```python
from build123d import *

# Parameters (mm, degrees)
SKETCH1_R           = 3.5
BOSS_EXTRUDE1_DEPTH = 60
BOSS_EXTRUDE2_DEPTH = 5
BOSS_EXTRUDE3_START = 5
SKETCH1_4_R         = 1.25
SKETCH1_4_R_2       = 2.143
BOSS_EXTRUDE3_DEPTH = 3
CUT_EXTRUDE1_REACH  = 213.819
BOSS_EXTRUDE4_START = 57
SKETCH1_6_R         = 3.5
SKETCH1_6_R_2       = 1.8
BOSS_EXTRUDE4_DEPTH = 3


with BuildPart() as part:
    # Sketch1 → Boss-Extrude1 (new body)
    with BuildSketch(Plane(origin=(0, 0, 0), x_dir=(1, 0, 0), z_dir=(0, 1, 0))):
        with BuildLine():
            ThreePointArc((0, 58.25), (17.061029996, 17.061029996), (58.25, 0))
            Line((58.25, 0), (118.99047, 0))
            ThreePointArc((118.99047, 0), (137.127758937, 7.512711063), (144.64047, 25.65))
            Line((144.64047, 25.65), (144.64047, 86.39047))
            ThreePointArc((144.64047, 86.39047), (127.579440004, 127.579440004), (86.39047, 144.64047))
            Line((86.39047, 144.64047), (58.25, 144.64047))
            ThreePointArc((58.25, 144.64047), (17.061029996, 127.579440004), (0, 86.39047))
            Line((0, 86.39047), (0, 58.25))
        make_face()
        with Locations(Location((66.320235, 6, 0), (0, 0, 270))):
            Circle(SKETCH1_R, mode=Mode.SUBTRACT)
        with BuildLine():
            ThreePointArc((5, 86.39047), (20.596563902, 124.043906098), (58.25, 139.64047))
            Line((58.25, 139.64047), (72.320235, 139.64047))
            Line((72.320235, 139.64047), (72.320235, 138.64047))
            ThreePointArc((72.320235, 138.64047), (78.320235, 132.64047), (84.320235, 138.64047))
            Line((84.320235, 138.64047), (84.320235, 139.600211843))
            ThreePointArc((84.320235, 139.600211843), (123.304711738, 124.768865705), (139.64047, 86.39047))
            Line((139.64047, 86.39047), (139.64047, 72.320235))
            Line((139.64047, 72.320235), (138.64047, 72.320235))
            ThreePointArc((138.64047, 72.320235), (132.64047, 66.320235), (138.64047, 60.320235))
            Line((138.64047, 60.320235), (139.64047, 60.320235))
            Line((139.64047, 60.320235), (139.64047, 25.65))
            ThreePointArc((139.64047, 25.65), (133.592225032, 11.048244968), (118.99047, 5))
            Line((118.99047, 5), (101.050235, 5))
            Line((101.050235, 5), (101.050235, 4.54))
            Line((101.050235, 4.54), (101.050235, 2))
            Line((101.050235, 2), (100.050235, 2))
            Line((100.050235, 2), (93.970235, 2))
            Line((93.970235, 2), (83.270235, 2))
            Line((83.270235, 2), (77.190235, 2))
            Line((77.190235, 2), (76.190235, 2))
            Line((76.190235, 2), (76.190235, 4.54))
            Line((76.190235, 4.54), (76.190235, 5))
            Line((76.190235, 5), (72.320235, 5))
            Line((72.320235, 5), (72.320235, 6))
            ThreePointArc((72.320235, 6), (66.320235, 12), (60.320235, 6))
            Line((60.320235, 6), (60.320235, 5))
            Line((60.320235, 5), (58.25, 5))
            ThreePointArc((58.25, 5), (20.596563902, 20.596563902), (5, 58.25))
            Line((5, 58.25), (5, 72.320235))
            Line((5, 72.320235), (6, 72.320235))
            ThreePointArc((6, 72.320235), (12, 78.320235), (6, 84.320235))
            Line((6, 84.320235), (5, 84.320235))
            Line((5, 84.320235), (5, 86.39047))
        make_face(mode=Mode.SUBTRACT)
        with Locations(Location((138.64047, 66.320235, 0), (0, 0, 270))):
            Circle(SKETCH1_R, mode=Mode.SUBTRACT)
        with Locations(Location((6, 78.320235, 0), (0, 0, 270))):
            Circle(SKETCH1_R, mode=Mode.SUBTRACT)
        with Locations(Location((78.320235, 138.64047, 0), (0, 0, 270))):
            Circle(SKETCH1_R, mode=Mode.SUBTRACT)
    extrude(amount=BOSS_EXTRUDE1_DEPTH)

    # Sketch1<2> → Boss-Extrude2 (add)
    with BuildSketch(Plane(origin=(0, 0, 0), x_dir=(1, 0, 0), z_dir=(0, 1, 0))):
        with BuildLine():
            Line((72.320235, 139.64047), (58.25, 139.64047))
            ThreePointArc((58.25, 139.64047), (20.596563902, 124.043906098), (5, 86.39047))
            Line((5, 86.39047), (5, 84.320235))
            Line((5, 84.320235), (6, 84.320235))
            ThreePointArc((6, 84.320235), (12, 78.320235), (6, 72.320235))
            Line((6, 72.320235), (5, 72.320235))
            Line((5, 72.320235), (5, 58.25))
            ThreePointArc((5, 58.25), (20.596563902, 20.596563902), (58.25, 5))
            Line((58.25, 5), (60.320235, 5))
            Line((60.320235, 5), (60.320235, 6))
            ThreePointArc((60.320235, 6), (66.320235, 12), (72.320235, 6))
            Line((72.320235, 6), (72.320235, 5))
            Line((72.320235, 5), (76.190235, 5))
            Line((76.190235, 5), (76.190235, 2))
            Line((76.190235, 2), (101.050235, 2))
            Line((101.050235, 2), (101.050235, 5))
            Line((101.050235, 5), (118.99047, 5))
            ThreePointArc((118.99047, 5), (133.592225032, 11.048244968), (139.64047, 25.65))
            Line((139.64047, 25.65), (139.64047, 60.320235))
            Line((139.64047, 60.320235), (138.64047, 60.320235))
            ThreePointArc((138.64047, 60.320235), (132.64047, 66.320235), (138.64047, 72.320235))
            Line((138.64047, 72.320235), (139.64047, 72.320235))
            Line((139.64047, 72.320235), (139.64047, 86.39047))
            ThreePointArc((139.64047, 86.39047), (123.304711738, 124.768865705), (84.320235, 139.600211843))
            Line((84.320235, 139.600211843), (84.320235, 138.64047))
            ThreePointArc((84.320235, 138.64047), (78.320235, 132.64047), (72.320235, 138.64047))
            Line((72.320235, 138.64047), (72.320235, 139.64047))
        make_face()
    extrude(amount=BOSS_EXTRUDE2_DEPTH)

    # Sketch1<4> → Boss-Extrude3 (add)
    # profile 1 of 4: a face of its own
    with BuildSketch(Plane(origin=(0, 0, 0), x_dir=(1, 0, 0), z_dir=(0, 1, 0)).offset(BOSS_EXTRUDE3_START)):
        with BuildLine():
            Line((101.050235, 2), (101.050235, 4.54))
            ThreePointArc((101.050235, 4.54), (97.510235, 8.08), (93.970235, 4.54))
            Line((93.970235, 4.54), (93.970235, 2))
            Line((93.970235, 2), (101.050235, 2))
        make_face()
        with Locations(Location((97.510235, 4.54, 0), (0, 0, 270))):
            Circle(SKETCH1_4_R, mode=Mode.SUBTRACT)
    # profile 2 of 4: a face of its own
    with BuildSketch(Plane(origin=(0, 0, 0), x_dir=(1, 0, 0), z_dir=(0, 1, 0)).offset(BOSS_EXTRUDE3_START)):
        with BuildLine():
            ThreePointArc((83.270235, 4.54), (79.730235, 8.08), (76.190235, 4.54))
            Line((76.190235, 4.54), (76.190235, 2))
            Line((76.190235, 2), (83.270235, 2))
            Line((83.270235, 2), (83.270235, 4.54))
        make_face()
        with Locations(Location((79.730235, 4.54, 0), (0, 0, 270))):
            Circle(SKETCH1_4_R, mode=Mode.SUBTRACT)
    # profile 3 of 4: a face of its own
    with BuildSketch(Plane(origin=(0, 0, 0), x_dir=(1, 0, 0), z_dir=(0, 1, 0)).offset(BOSS_EXTRUDE3_START)):
        with Locations(Location((79.730235, 50.26, 0), (0, 0, 270))):
            Circle(SKETCH1_4_R_2)
    # profile 4 of 4: a face of its own
    with BuildSketch(Plane(origin=(0, 0, 0), x_dir=(1, 0, 0), z_dir=(0, 1, 0)).offset(BOSS_EXTRUDE3_START)):
        with Locations(Location((97.510235, 50.26, 0), (0, 0, 270))):
            Circle(SKETCH1_4_R_2)
    extrude(amount=BOSS_EXTRUDE3_DEPTH)

    # Sketch2 → Cut-Extrude1 (cut, up to next)
    with BuildSketch(Plane(origin=(0, 0, -2), x_dir=(-1, 0, 0), z_dir=(0, 0, -1)), mode=Mode.PRIVATE) as cut_extrude1_sk1:
        with BuildLine():
            Line((-91.840235, 13.4), (-85.400235, 13.4))
            ThreePointArc((-85.400235, 13.4), (-84.092087455, 12.858147545), (-83.550235, 11.55))
            Line((-83.550235, 11.55), (-83.550235, 10.84))
            ThreePointArc((-83.550235, 10.84), (-84.092087455, 9.531852455), (-85.400235, 8.99))
            Line((-85.400235, 8.99), (-91.840235, 8.99))
            ThreePointArc((-91.840235, 8.99), (-93.148382545, 9.531852455), (-93.690235, 10.84))
            Line((-93.690235, 10.84), (-93.690235, 11.55))
            ThreePointArc((-93.690235, 11.55), (-93.148382545, 12.858147545), (-91.840235, 13.4))
        make_face()
    cut_extrude1_tool1 = extrude(cut_extrude1_sk1.sketch, amount=-CUT_EXTRUDE1_REACH, mode=Mode.PRIVATE) & part.part
    add(cut_extrude1_tool1.solids().sort_by_distance((88.620235, 11.195, -2))[0], mode=Mode.SUBTRACT)

    # Sketch1<6> → Boss-Extrude4 (add)
    # profile 1 of 4: a face of its own
    with BuildSketch(Plane(origin=(0, 0, 0), x_dir=(1, 0, 0), z_dir=(0, 1, 0)).offset(BOSS_EXTRUDE4_START)):
        with Locations(Location((6, 78.320235, 0), (0, 0, 270))):
            Circle(SKETCH1_6_R)
        with Locations(Location((6, 78.320235, 0), (0, 0, 270))):
            Circle(SKETCH1_6_R_2, mode=Mode.SUBTRACT)
    # profile 2 of 4: a face of its own
    with BuildSketch(Plane(origin=(0, 0, 0), x_dir=(1, 0, 0), z_dir=(0, 1, 0)).offset(BOSS_EXTRUDE4_START)):
        with Locations(Location((78.320235, 138.64047, 0), (0, 0, 270))):
            Circle(SKETCH1_6_R)
        with Locations(Location((78.320235, 138.64047, 0), (0, 0, 270))):
            Circle(SKETCH1_6_R_2, mode=Mode.SUBTRACT)
    # profile 3 of 4: a face of its own
    with BuildSketch(Plane(origin=(0, 0, 0), x_dir=(1, 0, 0), z_dir=(0, 1, 0)).offset(BOSS_EXTRUDE4_START)):
        with Locations(Location((138.64047, 66.320235, 0), (0, 0, 270))):
            Circle(SKETCH1_6_R)
        with Locations(Location((138.64047, 66.320235, 0), (0, 0, 270))):
            Circle(SKETCH1_6_R_2, mode=Mode.SUBTRACT)
    # profile 4 of 4: a face of its own
    with BuildSketch(Plane(origin=(0, 0, 0), x_dir=(1, 0, 0), z_dir=(0, 1, 0)).offset(BOSS_EXTRUDE4_START)):
        with Locations(Location((66.320235, 6, 0), (0, 0, 270))):
            Circle(SKETCH1_6_R)
        with Locations(Location((66.320235, 6, 0), (0, 0, 270))):
            Circle(SKETCH1_6_R_2, mode=Mode.SUBTRACT)
    extrude(amount=BOSS_EXTRUDE4_DEPTH)


solid = part.part
```
Read the model definition and answer for the solid it produces. Units are mm, in the model's axes. A direction names the side the tool comes from. Coordinates: 2 decimals unless noted, no trailing zeros. Write each loop counter-clockwise with the first axis right and the second up, starting at its lowest first coordinate (ties: lowest second). Pieces come first, ordered by that corner, then holes. Notation, with made-up numbers: (65, -3.5) -> (69, -3.5) arc R23 cw to (69, 6.5) -> close; hole circle Ø4 at (26, 84). An arc over 180 degrees is marked (long way). Return JSON: item names as keys, results as strings.
1. A cutting plane is placed at A-A (z = -94). Determine the outline of the cut face in (x, y).
Found:
{"outline": "(0.5, 0) -> (144.14, 0) -> (144.14, 60) -> (139.09, 60) -> (139.09, 5) -> (5.55, 5) -> (5.55, 60) -> (0.5, 60) -> close"}
2. Find the intervals of material crossed by line 1 along Z through (x, y) = (75.5, 19); line 2 along X through (y, z) = (44.5, -79.5); line 3 along Y through (x, z) = (60, -43.5), in increasing order. Write a range as from..to.
Found:
{"line 1": "-144.64..-140.71, -136.57..-133.34, -5..0", "line 2": "0..2.7, 9.3..11.88, 139.64..144.64", "line 3": "0..5"}
3. A cutting plane is placed at D-D (z = -113.5). Determine the outline of the cut face in (x, y).
Found:
{"outline": "(6.69, 0) -> (137.95, 0) -> (137.95, 60) -> (132.22, 60) -> (132.22, 5) -> (12.42, 5) -> (12.42, 60) -> (6.69, 60) -> close"}
4. A cutting plane is placed at B-B (y = 20.5). Give the number of separate pieces and of enclosed holes in the cut face, and give its area (3 significant figures).
Found:
{"separate pieces": "1", "enclosed holes": "5", "area": "2,430 mm2"}
5. Determine the mould class of faces 4 (the face through (71, 0, -73)), 5 (the face through (128.03, 29.58, -127.124)), 6 (the face through (68.105, 58.479, -6.234)) for opening direction X: pulls with the +X half, pulls with the -X half, needs draft (parallel to the pull), parting line crosses it, or undercut.
Found:
{"face 4": "needs draft", "face 5": "pulls with the +X half", "face 6": "undercut"}
6. Each of these flat-tipped pins is pushed along its axis until it touches: P1, Ø2, axis at x = 79.73, z = -4.54, coming from the +Y side; P2, Ø17.5, axis at y = 40, z = -48.5, coming from the -X side; P3, Ø2, axis at x = 45, y = 21, coming from the +Z side. Where does it stop, or does it pass through?
Found:
{"P1": "y = 5", "P2": "x = 0.01", "P3": "z = -1.3"}
7. A tool of negligible diameter and unlimited length cuts with its end or side. For faces 1 (the face through (6.08, 58.48, -80.12)), 2 (the face through (77, 57, -137)), 3 (the face through (20.185, 32.115, -123.628)), from which of +Z, -Z, +X, -X, +Y, -Y can it reach the whole face along a straight path? Write none if from no direction.
Found:
{"face 1": "+Y, -Y", "face 2": "-Y", "face 3": "+Y"}
8. A cutting plane is placed at C-C (z = -50.26). Determine the outline of the cut face in (x, y), and give its area (3 significant figures).
Found:
{"outline": "(0.55, 0) -> (144.64, 0) -> (144.64, 60) -> (139.64, 60) -> (139.64, 5) -> (99.65, 5) -> (99.65, 8) -> (95.37, 8) -> (95.37, 5) -> (81.87, 5) -> (81.87, 8) -> (77.59, 8) -> (77.59, 5) -> (5.6, 5) -> (5.6, 60) -> (0.55, 60) -> close", "area": "1,300 mm2"}
